The drawing under review shows one solid part. Ordinate dimensions are in mm from its lowest x, y, z. Coordinates: 2 decimals unless noted, no trailing zeros. Write each loop counter-clockwise with the first axis right and the second up, starting at its lowest first coordinate (ties: lowest second). Pieces come first, ordered by that corner, then holes. Notation, with made-up numbers: M -5.5,-33 L 9.5,-33 A30 ccw 9.5,-11 Z; hole C 50,-17 d5. An arc over 180 degrees is marked long. Write item = value, one per line.
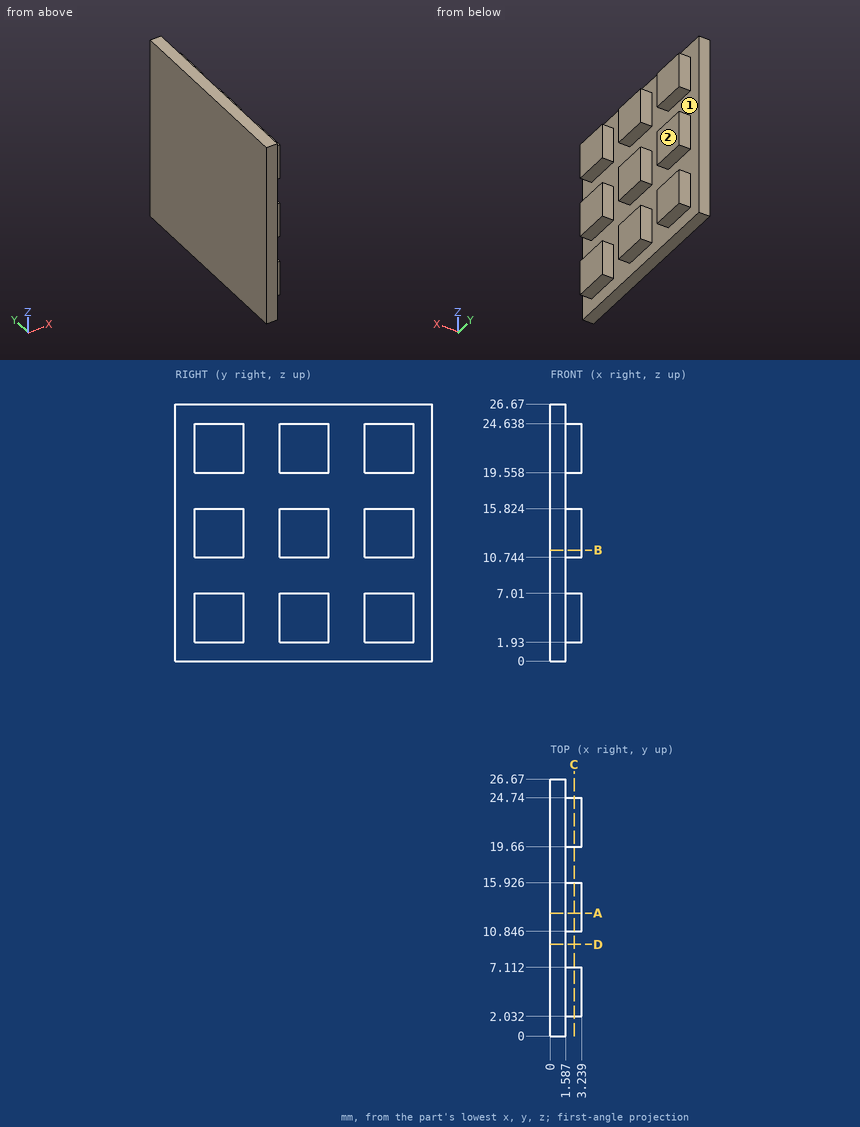
Q1. Consider section C-C, the plane x = 2.45. State how many separate pieces and enclosed holes the cut face has, and give its area (3 significant figures).
Check result:
separate_pieces = 9
enclosed_holes = 0
area = 232 mm²
Q2. Consider section B-B, the plane z = 11.5. State the section outline as (x, y) points (1 decimal).
Check result:
outline = M 0,0 L 1.6,0 L 1.6,2 L 3.2,2 L 3.2,7.1 L 1.6,7.1 L 1.6,10.8 L 3.2,10.8 L 3.2,15.9 L 1.6,15.9 L 1.6,19.7 L 3.2,19.7 L 3.2,24.7 L 1.6,24.7 L 1.6,26.7 L 0,26.7 Z
Q3. The part is to be moulded in two halves that separate along Z. For the marked faces 1 and 2, say which applies: +Z half, -Z half, draft (parallel to the pull), parting line (faces both ways), or undercut.
Check result:
face_1 = undercut
face_2 = draft
Q4. Consider section A-A, the plane y = 12.75. State the section outline as (x, z) points (1 decimal).
Check result:
outline = M 0,0 L 1.6,0 L 1.6,1.9 L 3.2,1.9 L 3.2,7 L 1.6,7 L 1.6,10.7 L 3.2,10.7 L 3.2,15.8 L 1.6,15.8 L 1.6,19.6 L 3.2,19.6 L 3.2,24.6 L 1.6,24.6 L 1.6,26.7 L 0,26.7 Z
Q5. Consider section D-D, the plane y = 9.5. State the section outline as (x, z) points.
Check result:
outline = M 0,0 L 1.59,0 L 1.59,26.67 L 0,26.67 Z
Q6. Wall thickness on line 1 (Y direction, x = 2.95, z = 6.75) (1 decimal); line 2 (Z direction, x = 2.4, y = 15.75) (1 decimal); line 3 (X direction, y = 25.25, z = 10.75): over which ranges is each line inside the solid? List them lowest first.
Check result:
line_1 = 2 to 7.1, 10.8 to 15.9, 19.7 to 24.7
line_2 = 1.9 to 7, 10.7 to 15.8, 19.6 to 24.6
line_3 = 0 to 1.59
Q7. For P1, Ø1.3, axis at x = 2.5, y = 21.5, coming from the +Z side; P2, Ø1.3, axis at x = 2.5, y = 14, coming from the -Z side; P3, Ø1.3, axis at x = 2.5, z = 5, coming from the -Y side, all flat-tipped, find the tip position at first contact; note any pin that passes through.
Check result:
P1 = 24.64
P2 = 1.93
P3 = 2.03
